Drawing for the job (mm, zero at the part's lowest x, y, z). Coordinates: 2 decimals unless noted, no trailing zeros. Order: outer loops, then holes, each group sorted by start corner. A loop starts at its lowest first (then second) coordinate and runs counter-clockwise, first axis right, second up. Notation, with made-up numbers: (24, 53.25) -> (52, 53.25) arc R28 cw to (52, 81.25) -> close; hole circle Ø6 at (70.5, 89). An arc over 180 degrees is marked (long way). Write each question's results on one line, items separated by ' | '.
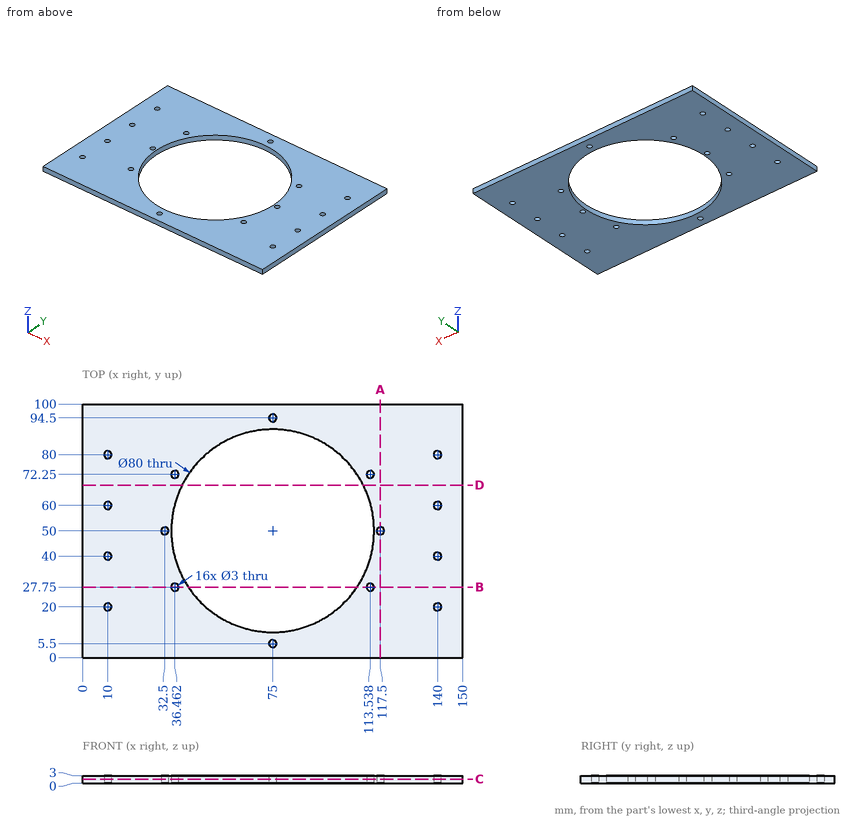
Item 1: Slice it at D-D, the plane y = 68. List the corners of the cut face in (x, z).
Answer:
outline: (0, 0) -> (39.28, 0) -> (39.28, 3) -> (0, 3) -> close; (110.72, 0) -> (150, 0) -> (150, 3) -> (110.72, 3) -> close
Item 2: Slice it at B-B, the plane y = 27.75. List the corners of the cut face in (x, z).
Answer:
outline: (0, 0) -> (34.96, 0) -> (34.96, 3) -> (0, 3) -> close; (37.96, 0) -> (41.76, 0) -> (41.76, 3) -> (37.96, 3) -> close; (108.24, 0) -> (112.04, 0) -> (112.04, 3) -> (108.24, 3) -> close; (115.04, 0) -> (150, 0) -> (150, 3) -> (115.04, 3) -> close
Item 3: Slice it at C-C, the plane z = 1.65. State how many separate pieces and enclosed holes the cut face has, and give its area (3 significant figures).
Answer:
separate pieces: 1 | enclosed holes: 17 | area: 9,860 mm^2
Item 4: Drill centre lines: line 1 (Y direction, x = 10, z = 1.7); line 2 (X direction, y = 94.5, z = 1.75); line 3 (X direction, y = 27, z = 2.6). Where is each one in solid material? Low to high. Write a range as from..to.
Answer:
line 1: y = 0..18.5, 21.5..38.5, 41.5..58.5, 61.5..78.5, 81.5..100 | line 2: x = 0..73.5, 76.5..150 | line 3: x = 0..35.16, 37.76..42.27, 107.73..112.24, 114.84..150
Item 5: Slice it at A-A, the plane x = 117.5. List the corners of the cut face in (y, z), and give its area (3 significant figures).
Answer:
outline: (0, 0) -> (48.5, 0) -> (48.5, 3) -> (0, 3) -> close; (51.5, 0) -> (100, 0) -> (100, 3) -> (51.5, 3) -> close | area: 291 mm^2
